Can you work these out from the drawing? Everything is in mm from the part's minimum corner. Give positions to 0.01 mm unless a question says otherwise; leave off trailing zeros. Loops run counter-clockwise (first coordinate to the right, second up) from the corner with the lowest first, then second, coordinate; pieces in that order, holes last.
Q1. I need wall thicknesses on line 1 (X direction, y = 0.25, z = 12.25) (3 decimals); line 2 (X direction, y = 1.65, z = 12.25) (3 decimals); line 3 (Z direction, x = 17, y = 1.6). Which ranges of each line are inside material? Lowest first, please.
Q2. If we section it at C-C (y = 1.3): Please give me the cut outline in (x, z) (3 decimals).
Q3. Will these pins go through, and if not, where does the flat tip stop? P1, Ø2.5, axis at x = 18, z = 12.25, coming from the +Y side; P2, Ø1.5, axis at x = 15.5, y = 1, coming from the -Z side.
Q4. If we section it at B-B (x = 12.25): Please give me the cut outline in (y, z) (3 decimals).
Q5. We'd pull the mould along X, two halves only. Please class the marked faces 1, 2 and 3: +X half, -X half, draft (parallel to the pull), parting line (faces both ways), or undercut.
Q6. If we section it at D-D (z = 9.5): Please give me the cut outline in (x, y).
Q7. If we section it at A-A (z = 12.25): Please give me the cut outline in (x, y) (3 decimals), plus the area to 3 significant figures.
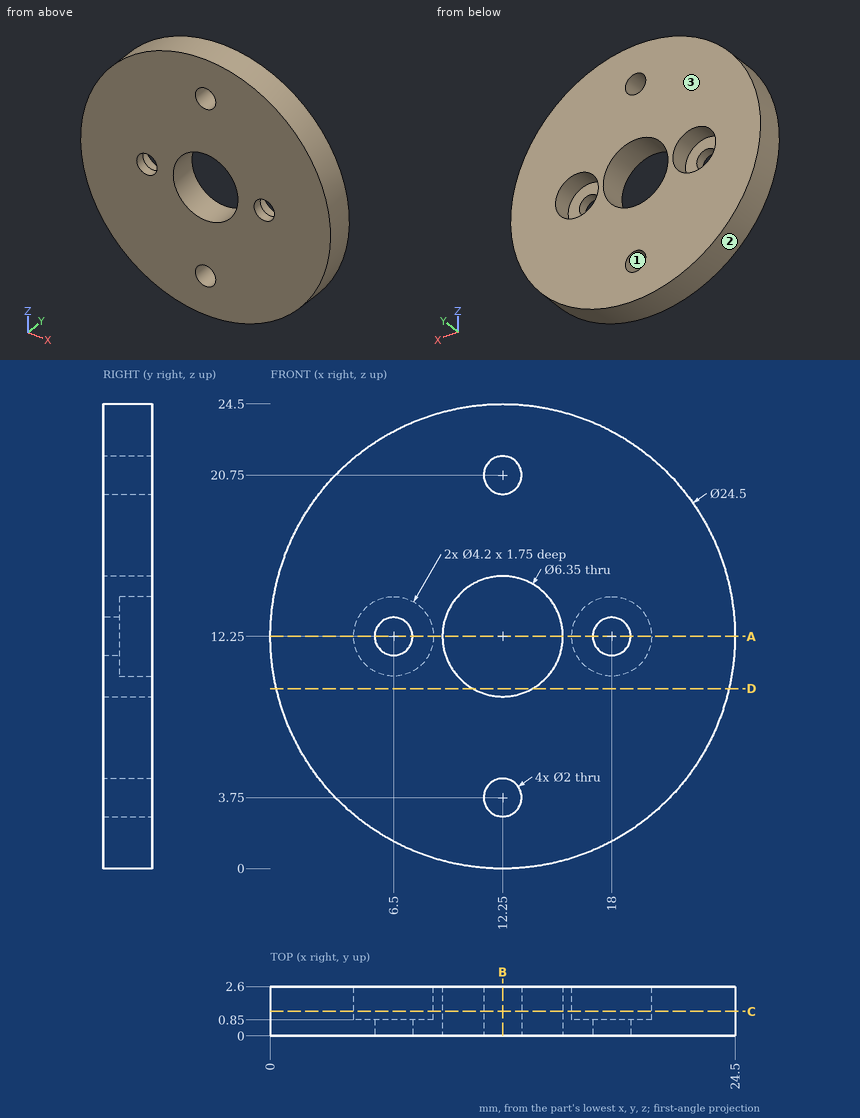
Check sheet entries:
1. line 1: x = 0 to 5.5, 7.5 to 9.075, 15.425 to 17, 19 to 24.5
1. line 2: x = 0 to 4.4, 8.6 to 9.075, 15.425 to 15.9, 20.1 to 24.5
1. line 3: z = 0.96 to 10.4, 14.1 to 23.54
2. outline: circle Ø24.5 at (12.25, 12.25); hole circle Ø4.2 at (6.5, 12.25); hole circle Ø6.35 at (12.25, 12.25); hole circle Ø2 at (12.25, 3.75); hole circle Ø2 at (12.25, 20.75); hole circle Ø4.2 at (18, 12.25)
3. P1: stops at y = 0.85
3. P2: stops at z = 0.26
4. outline: (0, 0) - (2.6, 0) - (2.6, 2.75) - (0, 2.75) - close; (0, 4.75) - (2.6, 4.75) - (2.6, 9.075) - (0, 9.075) - close; (0, 15.425) - (2.6, 15.425) - (2.6, 19.75) - (0, 19.75) - close; (0, 21.75) - (2.6, 21.75) - (2.6, 24.5) - (0, 24.5) - close
5. face 1: undercut
5. face 2: parting line
5. face 3: draft
6. outline: (0.31, 0) - (10.66, 0) - (10.66, 2.6) - (0.31, 2.6) - close; (13.84, 0) - (24.19, 0) - (24.19, 2.6) - (13.84, 2.6) - close
7. outline: (0, 0) - (5.5, 0) - (5.5, 0.85) - (4.4, 0.85) - (4.4, 2.6) - (0, 2.6) - close; (7.5, 0) - (9.075, 0) - (9.075, 2.6) - (8.6, 2.6) - (8.6, 0.85) - (7.5, 0.85) - close; (15.425, 0) - (17, 0) - (17, 0.85) - (15.9, 0.85) - (15.9, 2.6) - (15.425, 2.6) - close; (19, 0) - (24.5, 0) - (24.5, 2.6) - (20.1, 2.6) - (20.1, 0.85) - (19, 0.85) - close
7. area: 29.1 mm2
